from build123d import *

# Parameters (mm, degrees)
F0_W     = 228.6
F0_H     = 114.3
F1_DEPTH = 19.05
F2_R     = 38.1
F3_DEPTH = 25.4
F5_DEPTH = 25.4


with BuildPart() as f1:
    # F0 (on Front) → F1 (new body)
    with BuildSketch(Plane.XZ):
        with Locations((114.3, 57.15)):
            Rectangle(F0_W, F0_H)
    extrude(amount=F1_DEPTH)

    # F2 (on face) → F3 (cut)
    with BuildSketch(Plane.XZ.offset(19.05)):
        with Locations((47.625, 44.45)):
            Circle(F2_R)
        with Locations((180.975, 44.45)):
            Circle(F2_R)
    extrude(amount=-F3_DEPTH, mode=Mode.SUBTRACT)

    # F4 (on face) → F5 (cut)
    with BuildSketch(Plane.XZ.offset(19.05)):
        with BuildLine():
            ThreePointArc((152.571006, 69.843368), (165.414963, 79.227798), (180.971239, 82.55))
            Line((180.971239, 82.55), (141.666685, 82.54612))
            Line((141.666685, 82.54612), (141.666075, 88.724122))
            Line((141.666075, 88.724122), (152.4, 88.725182))
            Line((152.4, 88.725182), (152.4, 114.3))
            Line((152.4, 114.3), (69.85, 114.3))
            Line((69.85, 114.3), (69.852526, 88.717033))
            Line((69.852526, 88.717033), (113.794894, 88.721371))
            Line((113.794894, 88.721371), (113.795504, 82.543368))
            Line((113.795504, 82.543368), (48.622711, 82.536934))
            ThreePointArc((48.622711, 82.536934), (63.637392, 79.021857), (76.028994, 69.843368))
            Line((76.028994, 69.843368), (152.571006, 69.843368))
        make_face()
    extrude(amount=-F5_DEPTH, mode=Mode.SUBTRACT)


solid = f1.part
Part model, mm, in its own coordinate system. A direction names the side the tool comes from. Coordinates: 2 decimals unless noted, no trailing zeros. Loops run counter-clockwise (first coordinate to the right, second up) from the corner with the lowest first, then second, coordinate; pieces in that order, holes last. Notation, with made-up numbers: (56.5, -16.5) - (72.5, -16.5) arc R5 cw to (72.5, -10.5) - close; hole circle Ø10 at (-4, 57.25). An arc over 180 degrees is marked (long way). Write each question's results on one line, items separated by ' | '. Start each with the question number.
Q1. Probe line 1 along X through (y, z) = (-7.75, 44.45) (3 decimals); line 2 along Z through (x, y) = (107.5, -4.5); line 3 along X through (y, z) = (-1.75, 85.5). List the from-to ranges inside material, lowest first.
Q2. Slice it at A-A on z = 44.45. Give the cut face in (x, y) (3 decimals), and give its area (3 significant figures).
Q3. Drop a flat-ended pin along its axis: pin 1 Ø5.5 at (x, y) = (149.5, -5.5) entering from +Z. Give the stop position or say it passes through.
Q4. Slice it at B-B on x = 82.5. Give the cut face in (y, z).
Q5. Which spindle directions (+Z, -Z, +X, -X, +Y, -Y) get a long thin tool onto all of the face, cutting with end or side? Do faces 5 (the flat face through (113, -9, 0)), 6 (the flat face through (114, -10, 69.843)). Say none if no direction does.
Q6. Slice it at D-D on z = 105. Give the cut face in (x, y), and give its area (3 significant figures).
Q7. Slice it at C-C on x = 51.5. Give the cut face in (y, z).
Q8. Two-plate mould, pull along X, no slides. Class faces 1 (the flat face through (34, -9, 114.3)), 2 (the flat face through (152.4, -10, 101)), 3 (the flat face through (0, -9, 56)), 4 (the flat face through (228.6, -9, 56)): +X half, -X half, draft (parallel to the pull), parting line (faces both ways), or undercut.
Answer:
1) line 1: x = 0 to 9.525, 85.725 to 142.875, 219.075 to 228.6 | line 2: z = 0 to 69.84, 82.54 to 88.72 | line 3: x = 0 to 113.8, 141.67 to 228.6
2) outline: (0, -19.05) - (9.525, -19.05) - (9.525, 0) - (0, 0) - close; (85.725, -19.05) - (142.875, -19.05) - (142.875, 0) - (85.725, 0) - close; (219.075, -19.05) - (228.6, -19.05) - (228.6, 0) - (219.075, 0) - close | area: 1,450 mm2
3) pin 1: stops at z = 88.73
4) outline: (-19.05, 0) - (0, 0) - (0, 29.11) - (-19.05, 29.11) - close; (-19.05, 59.79) - (0, 59.79) - (0, 69.84) - (-19.05, 69.84) - close; (-19.05, 82.54) - (0, 82.54) - (0, 88.72) - (-19.05, 88.72) - close
5) face 5: -Z, +X, -X, +Y, -Y | face 6: +Y, -Y
6) outline: (0, -19.05) - (69.85, -19.05) - (69.85, 0) - (0, 0) - close; (152.4, -19.05) - (228.6, -19.05) - (228.6, 0) - (152.4, 0) - close | area: 2,780 mm2
7) outline: (-19.05, 0) - (0, 0) - (0, 6.55) - (-19.05, 6.55) - close; (-19.05, 82.54) - (0, 82.54) - (0, 114.3) - (-19.05, 114.3) - close
8) face 1: draft | face 2: undercut | face 3: -X half | face 4: +X half
